Model file for the job. Use its own axes, mm. A direction names the side the tool comes from. Coordinates: 2 decimals unless noted, no trailing zeros. Order: outer loops, then holes, each group sorted by start corner. A loop starts at its lowest first (then second) coordinate and runs counter-clockwise, first axis right, second up.
from build123d import *

# Parameters (mm, degrees)
SKETCH_1_W          = 60
SKETCH_1_H          = 88.5
SKETCH_1_R          = 2
EXTRUDE_1_DEPTH     = 3
SKETCH_2_R          = 12.675
CUT_EXTRUDE_1_DEPTH = 3
SKETCH_5_R          = 4.5
CUT_EXTRUDE_2_DEPTH = 10
EXTRUDE_2_DEPTH     = 3
SKETCH_7_W          = 60
SKETCH_7_H          = 8.4
EXTRUDE_3_DEPTH     = 3
CUT_EXTRUDE_3_DEPTH = 10
SKETCH_9_R          = 1.5
SKETCH_9_R_2        = 1.25
CUT_EXTRUDE_4_DEPTH = 62.867156068
SKETCH_10_W         = 14.9
SKETCH_10_H         = 3
EXTRUDE_4_DEPTH     = 3
SKETCH_11_R         = 1
CUT_EXTRUDE_5_DEPTH = 65.43946772
CHAMFER_1_SIZE      = 0.3
SKETCH_12_R         = 1.25
CUT_EXTRUDE_6_DEPTH = 65.43946772
FILLET_3_R          = 10
FILLET_4_R          = 1.75
FILLET_5_R          = 1.05
FILLET_6_R          = 1.25
CHAMFER_2_SIZE      = 1.5


with BuildPart() as part:
    # 草图1 → 凸台-拉伸1 (new body)
    with BuildSketch(Plane.XY):
        Rectangle(SKETCH_1_W, SKETCH_1_H)
        with Locations((25.11473671, 14.5)):
            Circle(SKETCH_1_R, mode=Mode.SUBTRACT)
        with Locations((0, -29)):
            Circle(SKETCH_1_R, mode=Mode.SUBTRACT)
        with Locations((-25.11473671, 14.5)):
            Circle(SKETCH_1_R, mode=Mode.SUBTRACT)
    extrude(amount=EXTRUDE_1_DEPTH)

    # 草图2 → 切除-拉伸1 (cut)
    with BuildSketch(Plane.XY.offset(3)):
        Circle(SKETCH_2_R)
    extrude(amount=-CUT_EXTRUDE_1_DEPTH, mode=Mode.SUBTRACT)

    # 草图5 → 切除-拉伸2 (cut)
    with BuildSketch(Plane.XY.offset(3)):
        with Locations((0, -19.25)):
            Circle(SKETCH_5_R)
        Polygon((-11.796598839, -10.967691454), (-15.796598839, -4.039488223), (-20.646341101, -6.839488223), (-16.646341101, -13.767691454), align=None)
    extrude(amount=-CUT_EXTRUDE_2_DEPTH, mode=Mode.SUBTRACT)

    # 草图6 → 凸台-拉伸2 (add)
    with BuildSketch(Plane.XY.offset(3)):
        with BuildLine():
            ThreePointArc((-30, 12.104647868), (-32.35, 0), (-30, -12.104647868))
            Line((-30, -12.104647868), (-30, 12.104647868))
        make_face()
        with BuildLine():
            Line((30, -12.104647868), (30, 12.104647868))
            ThreePointArc((30, 12.104647868), (32.35, 0), (30, -12.104647868))
        make_face()
    extrude(amount=-EXTRUDE_2_DEPTH)

    # 草图7 → 凸台-拉伸3 (add)
    with BuildSketch(Plane(origin=(0, 0, 0), x_dir=(-1, 0, 0), z_dir=(0, 0, -1))):
        with Locations((0, 48.45)):
            Rectangle(SKETCH_7_W, SKETCH_7_H)
    extrude(amount=-EXTRUDE_3_DEPTH)

    # 草图8 → 切除-拉伸3 (cut)
    with BuildSketch(Plane(origin=(0, 0, 0), x_dir=(-1, 0, 0), z_dir=(0, 0, -1))):
        with BuildLine():
            Line((-24, 42.278197597), (-24, 23.156478575))
            ThreePointArc((-24, 23.156478575), (-20.689565781, 26.156535852), (-17.007848271, 28.687202673))
            Line((-17.007848271, 28.687202673), (-24, 42.278197597))
        make_face()
        Polygon((-13.456964392, 30.52877694), (-10.106820911, 46.65), (-21.750841208, 46.65), align=None)
        with BuildLine():
            ThreePointArc((-7.964394001, 32.385041735), (0, 33.35), (7.964394001, 32.385041735))
            Line((7.964394001, 32.385041735), (5, 46.65))
            Line((5, 46.65), (-5, 46.65))
            Line((-5, 46.65), (-7.964394001, 32.385041735))
        make_face()
        Polygon((13.456964392, 30.52877694), (21.750841208, 46.65), (10.106820911, 46.65), align=None)
        with BuildLine():
            ThreePointArc((17.007848271, 28.687202673), (20.689565781, 26.156535852), (24, 23.156478575))
            Line((24, 23.156478575), (24, 42.278197597))
            Line((24, 42.278197597), (17.007848271, 28.687202673))
        make_face()
        with BuildLine():
            Line((-11.261417029, -38.25), (2.514135631, -38.25))
            Line((2.514135631, -38.25), (1.862188411, -33.297969222))
            ThreePointArc((1.862188411, -33.297969222), (-3.630710276, -33.15177888), (-9.025046714, -32.105623056))
            Line((-9.025046714, -32.105623056), (-11.261417029, -38.25))
        make_face()
        with BuildLine():
            ThreePointArc((-13.723509818, -30.395522339), (-19.205903699, -27.264551401), (-24, -23.156478575))
            Line((-24, -23.156478575), (-24, -38.25))
            Line((-24, -38.25), (-16.582305892, -38.25))
            Line((-16.582305892, -38.25), (-13.723509818, -30.395522339))
        make_face()
        with BuildLine():
            Line((6.819412718, -32.645338261), (7.557280434, -38.25))
            Line((7.557280434, -38.25), (22.444276173, -38.25))
            Line((22.444276173, -38.25), (13.304838766, -30.581101442))
            ThreePointArc((13.304838766, -30.581101442), (10.114921792, -31.779094656), (6.819412718, -32.645338261))
        make_face()
        with BuildLine():
            Line((24, -36.944592711), (24, -23.156478575))
            ThreePointArc((24, -23.156478575), (19.911359511, -26.753696239), (15.291790802, -29.637537584))
            Line((15.291790802, -29.637537584), (24, -36.944592711))
        make_face()
    extrude(amount=-CUT_EXTRUDE_3_DEPTH, mode=Mode.SUBTRACT)

    # 草图9 → 切除-拉伸4 (cut, through all)
    with BuildSketch(Plane(origin=(0, 0, 0), x_dir=(-1, 0, 0), z_dir=(0, 0, -1))):
        with Locations((5, 49.65)):
            Circle(SKETCH_9_R)
        with Locations((-15, 49.65)):
            Circle(SKETCH_9_R)
        with Locations(Location((5, -41.25, 0), (0, 0, 180))):
            Circle(SKETCH_9_R)
        with Locations(Location((-15, -41.25, 0), (0, 0, 180))):
            Circle(SKETCH_9_R)
        with Locations((-27, -28.25)):
            Circle(SKETCH_9_R_2)
        with Locations(Location((-27, 36.65, 0), (0, 0, 180))):
            Circle(SKETCH_9_R_2)
    extrude(amount=-CUT_EXTRUDE_4_DEPTH, mode=Mode.SUBTRACT)

    # 草图10 → 凸台-拉伸4 (add)
    with BuildSketch(Plane(origin=(0, 0, 0), x_dir=(-1, 0, 0), z_dir=(0, 0, -1))):
        with Locations((-15.05, 54.15)):
            Rectangle(SKETCH_10_W, SKETCH_10_H)
        with Locations((15.05, 54.15)):
            Rectangle(SKETCH_10_W, SKETCH_10_H)
        with Locations((15.05, -45.75)):
            Rectangle(SKETCH_10_W, SKETCH_10_H)
        with Locations((-15.05, -45.75)):
            Rectangle(SKETCH_10_W, SKETCH_10_H)
    extrude(amount=-EXTRUDE_4_DEPTH)

    # 草图11 → 切除-拉伸5 (cut, through all)
    with BuildSketch(Plane(origin=(0, 0, 0), x_dir=(-1, 0, 0), z_dir=(0, 0, -1))):
        with Locations((-23.5, 52.65)):
            Circle(SKETCH_11_R)
        with Locations((-6.6, 52.65)):
            Circle(SKETCH_11_R)
        with Locations((6.6, 52.65)):
            Circle(SKETCH_11_R)
        with Locations((23.5, 52.65)):
            Circle(SKETCH_11_R)
        with Locations((23.5, -44.25)):
            Circle(SKETCH_11_R)
        with Locations((6.6, -44.25)):
            Circle(SKETCH_11_R)
        with Locations((-6.6, -44.25)):
            Circle(SKETCH_11_R)
        with Locations((-23.5, -44.25)):
            Circle(SKETCH_11_R)
    extrude(amount=-CUT_EXTRUDE_5_DEPTH, mode=Mode.SUBTRACT)

    # 倒角1
    chamfer_1_edges = [part.edges().sort_by_distance(p)[0] for p in [
        (7.6, 55.65, 1.5),
        (22.5, 55.65, 1.5),
        (-7.6, 55.65, 1.5),
        (-22.5, 55.65, 1.5),
        (-7.6, -47.25, 1.5),
        (-22.5, -47.25, 1.5),
        (7.6, -47.25, 1.5),
        (22.5, -47.25, 1.5),
    ]]
    chamfer(chamfer_1_edges, length=CHAMFER_1_SIZE)

    # 草图12 → 切除-拉伸6 (cut, through all)
    with BuildSketch(Plane(origin=(0, 0, 0), x_dir=(-1, 0, 0), z_dir=(0, 0, -1))):
        with Locations((-9, 15.588457268)):
            Circle(SKETCH_12_R)
        with Locations((18, 0)):
            Circle(SKETCH_12_R)
        with Locations((-9, -15.588457268)):
            Circle(SKETCH_12_R)
    extrude(amount=-CUT_EXTRUDE_6_DEPTH, mode=Mode.SUBTRACT)

    # 圆角3
    fillet_3_edges = [part.edges().sort_by_distance(p)[0] for p in [
        (-30, 12.104647868, 1.5),
        (-30, -12.104647868, 1.5),
        (30, -12.104647868, 1.5),
        (30, 12.104647868, 1.5),
    ]]
    fillet(fillet_3_edges, radius=FILLET_3_R)

    # 圆角4
    fillet_4_edges = [part.edges().sort_by_distance(p)[0] for p in [
        (-6.819412718, -32.645338261, 1.5),
        (-13.304838766, -30.581101442, 1.5),
        (-7.557280434, -38.25, 1.5),
        (-15.291790802, -29.637537584, 1.5),
        (-24, -23.156478575, 1.5),
        (24, -23.156478575, 1.5),
        (13.723509818, -30.395522339, 1.5),
        (16.582305892, -38.25, 1.5),
        (24, -38.25, 1.5),
        (9.025046714, -32.105623056, 1.5),
        (-1.862188411, -33.297969222, 1.5),
        (-2.514135631, -38.25, 1.5),
        (11.261417029, -38.25, 1.5),
        (-10.106820911, 46.65, 1.5),
        (-21.750841208, 46.65, 1.5),
        (-13.456964392, 30.52877694, 1.5),
        (-24, 23.156478575, 1.5),
        (-17.007848271, 28.687202673, 1.5),
        (-7.964394001, 32.385041735, 1.5),
        (7.964394001, 32.385041735, 1.5),
        (5, 46.65, 1.5),
        (-5, 46.65, 1.5),
        (10.106820911, 46.65, 1.5),
        (13.456964392, 30.52877694, 1.5),
        (21.750841208, 46.65, 1.5),
        (17.007848271, 28.687202673, 1.5),
        (24, 23.156478575, 1.5),
    ]]
    fillet(fillet_4_edges, radius=FILLET_4_R)

    # 圆角5
    fillet_5_edges = [part.edges().sort_by_distance(p)[0] for p in [
        (-16.646341101, -13.767691454, 1.5),
        (-20.646341101, -6.839488223, 1.5),
        (-15.796598839, -4.039488223, 1.5),
        (-11.796598839, -10.967691454, 1.5),
    ]]
    fillet(fillet_5_edges, radius=FILLET_5_R)

    # 圆角6
    fillet_6_edges = [part.edges().sort_by_distance(p)[0] for p in [
        (-22.444276173, -38.25, 1.5),
        (-24, -36.944592711, 1.5),
        (-24, 42.278197597, 1.5),
        (24, 42.278197597, 1.5),
    ]]
    fillet(fillet_6_edges, radius=FILLET_6_R)

    # 倒角2
    chamfer_2_edges = [part.edges().sort_by_distance(p)[0] for p in [
        (10.25, 15.588457268, 0),
        (-16.75, 0, 0),
        (10.25, -15.588457268, 0),
    ]]
    chamfer(chamfer_2_edges, length=CHAMFER_2_SIZE)


solid = part.part
Q1. Which spindle directions (+Z, -Z, +X, -X, +Y, -Y) get a long thin tool onto all of the face, cutting with end or side? Do faces 1 (the face through (0, -44.25, 1)), 2 (the face through (19.786, 26.847, 1.479)), 3 (the face through (-15, -47.25, 1)), 4 (the face through (7.6, 54, 1)). Say none if no direction does.
Established:
face 1: +Z, -Z, -Y
face 2: +Z, -Z
face 3: +Z, -Z, +X, -X, -Y
face 4: +Z, -Z, +Y
Q2. Cut at C-C, the plane z = 2.45. Count the separate pieces of the cut face and the enclosed holes in it, plus the area to 3 significant figures.
Established:
separate pieces: 1
enclosed holes: 24
area: 4,620 mm2
Q3. Cut at B-B, the plane y = 22.5. List the corners of the cut face in (x, z), plus the area to 3 significant figures.
Established:
outline: (-30, 0) - (30, 0) - (30, 3) - (-30, 3) - close
area: 180 mm2
Q4. Drop flat-ended pins along their axis: P1, Ø1.5, axis at x = 1, z = 1.5, coming from the -Y side; P2, Ø1.5, axis at y = -29, z = 2, coming from the +X side; P3, Ø0.8, axis at y = -45, z = 1, coming from the -X side. Give the stop position or say it passes through.
Established:
P1: stops at y = -44.25
P2: stops at x = 30
P3: stops at x = -22.5
Q5. Cut at A-A, the plane y = 6.5. List the corners of the cut face in (x, z), plus the area to 3 significant figures.
Established:
outline: (-31.69, 0) - (-10.88, 0) - (-10.88, 3) - (-31.69, 3) - close; (10.88, 0) - (31.69, 0) - (31.69, 3) - (10.88, 3) - close
area: 125 mm2
Q6. Probe line 1 (Y direction, x = 0, z = 2.4) (3 decimals); line 2 (X direction, y = 29.5, z = 1.7); line 3 (Y direction, x = -5, z = 2.1). List the from-to ranges inside material, lowest first.
Established:
line 1: y = -44.25 to -38.25, -33.35 to -31, -27 to -23.75, -14.75 to -12.675, 12.675 to 33.35, 46.65 to 52.65
line 2: x = -30 to -24, -17.56 to 17.56, 24 to 30
line 3: y = -44.25 to -42.75, -39.75 to -11.65, 11.65 to 32.97, 45.92 to 48.15, 51.15 to 52.65
Q7. Mould opens along Y. For faces 5 (the face through (-0.59, -14.79, 1.52)), 6 (the face through (30, 33, 1)), 7 (the face through (27, 52.65, 1)) say: pulls with the +Y half, pulls with the -Y half, needs draft (parallel to the pull), parting line crosses it, or undercut.
Established:
face 5: undercut
face 6: needs draft
face 7: pulls with the +Y half
